Geometry check sheet. Reference: the model listing, model coordinates, mm. Face numbers are marked on the shaded views. Round coordinates to 2 decimals unless told otherwise and drop trailing zeros. Write each loop counter-clockwise with the first axis right and the second up, starting at its lowest first coordinate (ties: lowest second). Pieces come first, ordered by that corner, then holes.
Item 1: Cross-section at A-A (z = 16). Enter the section's corners in (x, y), then the cut area to 3 significant figures.
Item 2: Scan lines: probe 1 along X at (y, z) = (5, 20); probe 2 along X at (y, z) = (-12, 18); probe 3 along Y at (x, z) = (27.5, 18.5). Record each from-to range of solid material in increasing order.
Item 3: Draft check along X on the marked faces 1, 2 and 3. Enter one of: pulls with the +X half, pulls with the -X half, needs draft (parallel to the pull), parting line crosses it, or undercut.
Item 4: Depth check by flat-ended pin: P1, Ø6, axis at x = -8.5, z = 20, coming from the +Y side; P2, Ø3, axis at x = -24.5, y = 6, coming from the -Z side; P3, Ø2, axis at x = -13, y = -27, coming from the +Z side; P4, Ø3, axis at y = 18, z = 5, coming from the -X side. Enter the tip coordinate at first touch or a pass-through.
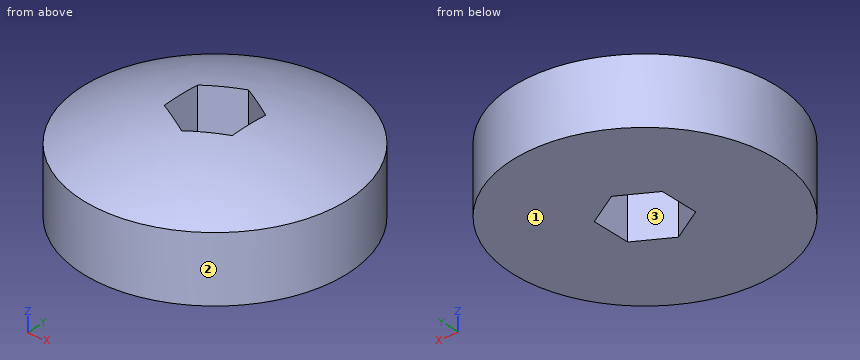
from build123d import *

# Parameters (mm, degrees)
F0_R     = 50
F1_DEPTH = 25
F4_DEPTH = 12.4837433515


with BuildPart() as f1:
    # F0 (on Top) → F1 (new body)
    with BuildSketch(Plane.XY):
        Circle(F0_R)
        Polygon((-12.9903810568, 7.5), (0, 15), (12.9903810568, 7.5), (12.9903810568, -7.5), (0, -15), (-12.9903810568, -7.5), align=None, mode=Mode.SUBTRACT)
    extrude(amount=F1_DEPTH)

    # F2 (on Front) → F3 (revolve)
    with BuildSketch(Plane.XZ):
        with BuildLine():
            Line((0, 25), (50, 25))
            ThreePointArc((50, 25), (25.7045802551, 34.0635888294), (0, 37.4827432515))
            Line((0, 37.4827432515), (0, 25))
        make_face()
    revolve(axis=Axis((0, 0, 31.2413716258), (0, 0, 1)))

    # F4 (cut, through all): a face of the model
    f4_faces = [f1.faces().sort_by_distance(p)[0] for p in [
        (0, 0, 25),
    ]]
    extrude(f4_faces, amount=-F4_DEPTH, mode=Mode.SUBTRACT)


solid = f1.part
Resolved:
1. outline: circle Ø100 at (0, 0); hole (-12.99, -7.5) - (0, -15) - (12.99, -7.5) - (12.99, 7.5) - (0, 15) - (-12.99, 7.5) - close
1. area: 7,270 mm2
2. probe 1: x = -49.75 to -12.99, 12.99 to 49.75
2. probe 2: x = -48.54 to -5.2, 5.2 to 48.54
2. probe 3: y = -41.76 to 41.76
3. face 1: needs draft
3. face 2: parting line crosses it
3. face 3: undercut
4. P1: stops at y = 49.7
4. P2: stops at z = 0
4. P3: stops at z = 33.2
4. P4: stops at x = -47.2
